Check sheet for the modelled part. Datum: model origin and axes. Units: mm. A direction names the side the tool comes from. Round coordinates to 2 decimals unless told otherwise and drop trailing zeros. Order: outer loops, then holes, each group sorted by start corner. A loop starts at its lowest first (then second) coordinate and runs counter-clockwise, first axis right, second up.
```python
from build123d import *

# Parameters (mm, degrees)
SKETCH1_R           = 2.5
BOSS_EXTRUDE2_DEPTH = 190


with BuildPart() as part:
    # Sketch1 → Boss-Extrude2 (new body)
    with BuildSketch(Plane.XY):
        with BuildLine():
            Line((10, -4.1), (10, -8.5))
            ThreePointArc((10, -8.5), (9.560660172, -9.560660172), (8.5, -10))
            Line((8.5, -10), (4.1, -10))
            Line((4.1, -10), (4.1, -9.5))
            Line((4.1, -9.5), (3.6, -9.5))
            Line((3.6, -9.5), (3.6, -8.2))
            Line((3.6, -8.2), (5.5, -8.2))
            Line((5.5, -8.2), (5.5, -6.560660172))
            Line((5.5, -6.560660172), (3.425126266, -4.485786438))
            ThreePointArc((3.425126266, -4.485786438), (2.776279568, -4.052240935), (2.010912703, -3.9))
            Line((2.010912703, -3.9), (-2.010912703, -3.9))
            ThreePointArc((-2.010912703, -3.9), (-2.776279568, -4.052240935), (-3.425126266, -4.485786438))
            Line((-3.425126266, -4.485786438), (-5.5, -6.560660172))
            Line((-5.5, -6.560660172), (-5.5, -8.2))
            Line((-5.5, -8.2), (-3.6, -8.2))
            Line((-3.6, -8.2), (-3.6, -9.5))
            Line((-3.6, -9.5), (-4.1, -9.5))
            Line((-4.1, -9.5), (-4.1, -10))
            Line((-4.1, -10), (-8.5, -10))
            ThreePointArc((-8.5, -10), (-9.560660172, -9.560660172), (-10, -8.5))
            Line((-10, -8.5), (-10, -4.1))
            Line((-10, -4.1), (-9.5, -4.1))
            Line((-9.5, -4.1), (-9.5, -3.6))
            Line((-9.5, -3.6), (-8.2, -3.6))
            Line((-8.2, -3.6), (-8.2, -5.5))
            Line((-8.2, -5.5), (-6.560660172, -5.5))
            Line((-6.560660172, -5.5), (-4.485786438, -3.425126266))
            ThreePointArc((-4.485786438, -3.425126266), (-4.052240935, -2.776279568), (-3.9, -2.010912703))
            Line((-3.9, -2.010912703), (-3.9, 2.010912703))
            ThreePointArc((-3.9, 2.010912703), (-4.052240935, 2.776279568), (-4.485786438, 3.425126266))
            Line((-4.485786438, 3.425126266), (-6.560660172, 5.5))
            Line((-6.560660172, 5.5), (-8.2, 5.5))
            Line((-8.2, 5.5), (-8.2, 3.6))
            Line((-8.2, 3.6), (-9.5, 3.6))
            Line((-9.5, 3.6), (-9.5, 4.1))
            Line((-9.5, 4.1), (-10, 4.1))
            Line((-10, 4.1), (-10, 8.5))
            ThreePointArc((-10, 8.5), (-9.560660172, 9.560660172), (-8.5, 10))
            Line((-8.5, 10), (-4.1, 10))
            Line((-4.1, 10), (-4.1, 9.5))
            Line((-4.1, 9.5), (-3.6, 9.5))
            Line((-3.6, 9.5), (-3.6, 8.2))
            Line((-3.6, 8.2), (-5.5, 8.2))
            Line((-5.5, 8.2), (-5.5, 6.560660172))
            Line((-5.5, 6.560660172), (-3.425126266, 4.485786438))
            ThreePointArc((-3.425126266, 4.485786438), (-2.776279568, 4.052240935), (-2.010912703, 3.9))
            Line((-2.010912703, 3.9), (2.010912703, 3.9))
            ThreePointArc((2.010912703, 3.9), (2.776279568, 4.052240935), (3.425126266, 4.485786438))
            Line((3.425126266, 4.485786438), (5.5, 6.560660172))
            Line((5.5, 6.560660172), (5.5, 8.2))
            Line((5.5, 8.2), (3.6, 8.2))
            Line((3.6, 8.2), (3.6, 9.5))
            Line((3.6, 9.5), (4.1, 9.5))
            Line((4.1, 9.5), (4.1, 10))
            Line((4.1, 10), (8.5, 10))
            ThreePointArc((8.5, 10), (9.560660172, 9.560660172), (10, 8.5))
            Line((10, 8.5), (10, 4.1))
            Line((10, 4.1), (9.5, 4.1))
            Line((9.5, 4.1), (9.5, 3.6))
            Line((9.5, 3.6), (8.2, 3.6))
            Line((8.2, 3.6), (8.2, 5.5))
            Line((8.2, 5.5), (6.560660172, 5.5))
            Line((6.560660172, 5.5), (4.485786438, 3.425126266))
            ThreePointArc((4.485786438, 3.425126266), (4.052240935, 2.776279568), (3.9, 2.010912703))
            Line((3.9, 2.010912703), (3.9, -2.010912703))
            ThreePointArc((3.9, -2.010912703), (4.052240935, -2.776279568), (4.485786438, -3.425126266))
            Line((4.485786438, -3.425126266), (6.560660172, -5.5))
            Line((6.560660172, -5.5), (8.2, -5.5))
            Line((8.2, -5.5), (8.2, -3.6))
            Line((8.2, -3.6), (9.5, -3.6))
            Line((9.5, -3.6), (9.5, -4.1))
            Line((9.5, -4.1), (10, -4.1))
        make_face()
        Circle(SKETCH1_R, mode=Mode.SUBTRACT)
    extrude(amount=BOSS_EXTRUDE2_DEPTH)


solid = part.part
```
Item 1: Go/stop test with flat-tipped pins: P1, Ø2, axis at y = -0.5, z = 60.5, coming from the -X side; P2, Ø0.6, axis at x = -9.5, z = 100.5, coming from the +Y side; P3, Ø1, axis at x = -2, z = 25.5, coming from the +Y side. Record where each tip stops, or that it passes through.
Answer:
P1: stops at x = -3.9
P2: stops at y = 9.83
P3: stops at y = 3.96
Item 2: Release check for a two-part mould opening along X. For faces 5 (the flat face through (0, -3.9, 94)), 6 (the flat face through (10, 6, 94)), 7 (the flat face through (6, 10, 94)) record: released by +X, released by -X, zero draft, split by the parting line, or undercut.
Answer:
face 5: undercut
face 6: released by +X
face 7: zero draft
Item 3: Access from +Z, -Z, +X, -X, +Y, -Y to the whole of each face (thin tool, end or side, straight path). Record for faces 1 (the flat face through (-3.9, 0, 94)), 2 (the flat face through (-10, -6, 94)), 3 (the flat face through (3.9, 0, 94)), 4 (the flat face through (0, 3.9, 94)).
Answer:
face 1: +Z, -Z, -X
face 2: +Z, -Z, -X, +Y, -Y
face 3: +Z, -Z, +X
face 4: +Z, -Z, +Y
Item 4: Scan lines: line 1 along Y through (x, z) = (0, 60); line 2 along X through (y, z) = (8.75, 54.5); line 3 along Y through (x, z) = (9.25, 32.5). Record each from-to range of solid material in increasing order.
Answer:
line 1: y = -3.9 to -2.5, 2.5 to 3.9
line 2: x = -9.98 to -3.6, 3.6 to 9.98
line 3: y = -9.8 to -3.6, 3.6 to 9.8
Item 5: Sectioned sample at A-A (y = 0). Record the cut outline in (x, z), and give its area (3 significant figures).
Answer:
outline: (-3.9, 0) - (-2.5, 0) - (-2.5, 190) - (-3.9, 190) - close; (2.5, 0) - (3.9, 0) - (3.9, 190) - (2.5, 190) - close
area: 532 mm2
